Can you work these out from the model? Positions are in its coordinate system, mm. Give positions to 0.01 mm unless a question says otherwise; leave off trailing zeros. Order: outer loops, then holes, each group sorted by start corner. A loop starts at its lowest first (then second) coordinate and runs counter-clockwise, first axis right, second up.
Item 1: I want a section at D-D, the plane x = -1. Write out the boundary of the cut face in (y, z) (3 decimals).
Item 2: If I drill on line 1 along Y through (x, z) = (44.45, 3.25) (1 decimal); line 2 along Y through (x, z) = (-38.1, 2.75) (1 decimal); line 3 along X through (y, z) = (-35.5, 3.25), over which ranges is the centre line in solid material (lowest first)?
Item 3: I want a section at B-B, the plane x = 44.45. Count the separate pieces of the cut face and the enclosed holes in it, then the cut area to 3 significant figures.
```python
from build123d import *

# Parameters (mm, degrees)
SKETCH1_W                   = 152.4
SKETCH1_H                   = 95.25
BOSS_EXTRUDE1_DEPTH         = 6.35
F_1_4_CLEARANCE_HOLE1_D     = 6.7564
TAP_DRILL_FOR_1_4_20_TAP1_D = 5.1054


with BuildPart() as part:
    # Sketch1 → Boss-Extrude1 (new, symmetric)
    with BuildSketch(Plane.XY):
        Rectangle(SKETCH1_W, SKETCH1_H)
    extrude(amount=BOSS_EXTRUDE1_DEPTH, both=True)

    # 1/4 Clearance Hole1 (through all)
    with Locations(Plane.XY.offset(6.35)):
        with Locations((-44.45, 41.275), (44.45, 41.275), (69.785060268, 15.875), (69.785060268, -9.525), (69.785060268, -34.925), (-69.785060268, 15.875), (-69.785060268, -9.525), (-69.785060268, -34.925)):
            Hole(F_1_4_CLEARANCE_HOLE1_D / 2)

    # Tap Drill for 1/4-20 Tap1 (through all)
    with Locations(Plane.XY.offset(6.35)):
        with Locations((-38.1, -33.9852), (38.1, -33.9852), (-44.45, -8.5852), (44.45, -8.5852), (0, 4.1148)):
            Hole(TAP_DRILL_FOR_1_4_20_TAP1_D / 2)


solid = part.part
```
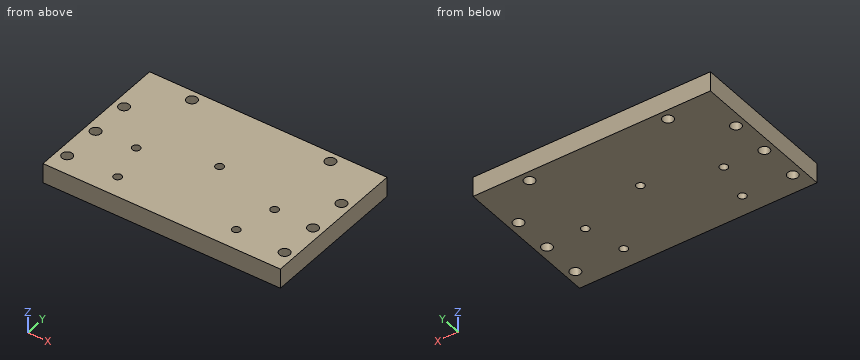
Results list:
1. outline: (-47.625, -6.35) - (1.766, -6.35) - (1.766, 6.35) - (-47.625, 6.35) - close; (6.463, -6.35) - (47.625, -6.35) - (47.625, 6.35) - (6.463, 6.35) - close
2. line 1: y = -47.6 to -11.1, -6 to 37.9, 44.7 to 47.6
2. line 2: y = -47.6 to -36.5, -31.4 to 47.6
2. line 3: x = -76.2 to -73.11, -66.46 to -40.15, -36.05 to 36.05, 40.15 to 66.46, 73.11 to 76.2
3. separate pieces: 3
3. enclosed holes: 0
3. area: 1,060 mm2
